```python
from build123d import *

# Parameters (mm, degrees)
SKETCH1_R           = 35
BOSS_EXTRUDE1_DEPTH = 12
SKETCH2_R           = 20.15
CUT_EXTRUDE1_DEPTH  = 5.5
SKETCH3_R           = 2.45
BOSS_EXTRUDE2_DEPTH = 5.5
SKETCH4_R           = 2.5
CUT_EXTRUDE2_DEPTH  = 50.922439844
SKETCH5_R           = 5.5
CUT_EXTRUDE3_DEPTH  = 5
SKETCH6_R           = 2.5
CUT_EXTRUDE4_DEPTH  = 51.931326313
CHAMFER1_SIZE       = 0.5
CHAMFER2_SIZE       = 0.5
CHAMFER3_SIZE       = 0.5


with BuildPart() as part:
    # Sketch1 → Boss-Extrude1 (new body)
    with BuildSketch(Plane(origin=(0, 0, 0), x_dir=(1, 0, 0), z_dir=(0, 1, 0))):
        with Locations(Location((0, 0, 0), (0, 0, 270))):
            Circle(SKETCH1_R)
    extrude(amount=BOSS_EXTRUDE1_DEPTH)

    # Sketch2 → Cut-Extrude1 (cut)
    with BuildSketch(Plane(origin=(0, 12, 0), x_dir=(1, 0, 0), z_dir=(0, 1, 0))):
        with Locations(Location((0, 0, 0), (0, 0, 270))):
            Circle(SKETCH2_R)
    extrude(amount=-CUT_EXTRUDE1_DEPTH, mode=Mode.SUBTRACT)

    # Sketch3 → Boss-Extrude2 (add)
    with BuildSketch(Plane(origin=(0, 6.5, 0), x_dir=(1, 0, 0), z_dir=(0, 1, 0))):
        with Locations(Location((0, -15.75, 0), (0, 0, 270))):
            Circle(SKETCH3_R)
    extrude(amount=BOSS_EXTRUDE2_DEPTH)

    # Sketch4 → Cut-Extrude2 (cut, through all)
    with BuildSketch(Plane(origin=(0, 6.5, 0), x_dir=(1, 0, 0), z_dir=(0, 1, 0))):
        with Locations(Location((11.136931804, 11.136931804, 0), (0, 0, 270))):
            Circle(SKETCH4_R)
        with Locations(Location((11.136931804, -11.136931804, 0), (0, 0, 270))):
            Circle(SKETCH4_R)
        with Locations(Location((-11.136931804, -11.136931804, 0), (0, 0, 270))):
            Circle(SKETCH4_R)
        with Locations(Location((-11.136931804, 11.136931804, 0), (0, 0, 270))):
            Circle(SKETCH4_R)
    extrude(amount=-CUT_EXTRUDE2_DEPTH, mode=Mode.SUBTRACT)

    # Sketch5 → Cut-Extrude3 (cut)
    with BuildSketch(Plane.XZ):
        with Locations(Location((11.136931804, -11.136931804, 0), (0, 0, 270))):
            Circle(SKETCH5_R)
        with Locations(Location((11.136931804, 11.136931804, 0), (0, 0, 270))):
            Circle(SKETCH5_R)
        with Locations(Location((-11.136931804, -11.136931804, 0), (0, 0, 270))):
            Circle(SKETCH5_R)
        with Locations(Location((-11.136931804, 11.136931804, 0), (0, 0, 270))):
            Circle(SKETCH5_R)
    extrude(amount=-CUT_EXTRUDE3_DEPTH, mode=Mode.SUBTRACT)

    # Sketch6 → Cut-Extrude4 (cut, through all)
    with BuildSketch(Plane.XZ):
        with Locations(Location((28.702, 0, 0), (0, 0, 270))):
            Circle(SKETCH6_R)
        with Locations(Location((20.295378834, -20.295378834, 0), (0, 0, 270))):
            Circle(SKETCH6_R)
        with Locations(Location((0, -28.702, 0), (0, 0, 270))):
            Circle(SKETCH6_R)
        with Locations(Location((-20.295378834, -20.295378834, 0), (0, 0, 270))):
            Circle(SKETCH6_R)
        with Locations(Location((-28.702, 0, 0), (0, 0, 270))):
            Circle(SKETCH6_R)
        with Locations(Location((-20.295378834, 20.295378834, 0), (0, 0, 270))):
            Circle(SKETCH6_R)
        with Locations(Location((0, 28.702, 0), (0, 0, 270))):
            Circle(SKETCH6_R)
        with Locations(Location((20.295378834, 20.295378834, 0), (0, 0, 270))):
            Circle(SKETCH6_R)
    extrude(amount=-CUT_EXTRUDE4_DEPTH, mode=Mode.SUBTRACT)

    # Chamfer1
    chamfer1_edges = [part.edges().sort_by_distance(p)[0] for p in [
        (0, 0, -35),
        (-11.136931804, 0, 16.636931804),
        (-11.136931804, 0, -5.636931804),
        (11.136931804, 0, -5.636931804),
        (11.136931804, 0, 16.636931804),
        (28.702, 0, 2.5),
        (20.295378834, 0, -17.795378834),
        (0, 0, -26.202),
        (-20.295378834, 0, -17.795378834),
        (-28.702, 0, 2.5),
        (-20.295378834, 0, 22.795378834),
        (0, 0, 31.202),
        (20.295378834, 0, 22.795378834),
    ]]
    chamfer(chamfer1_edges, length=CHAMFER1_SIZE)

    # Chamfer2
    chamfer2_edges = [part.edges().sort_by_distance(p)[0] for p in [
        (0, 12, -35),
        (0, 12, -20.15),
        (28.702, 12, 2.5),
        (20.295378834, 12, -17.795378834),
        (0, 12, -26.202),
        (-20.295378834, 12, -17.795378834),
        (-28.702, 12, 2.5),
        (-20.295378834, 12, 22.795378834),
        (0, 12, 31.202),
        (20.295378834, 12, 22.795378834),
    ]]
    chamfer(chamfer2_edges, length=CHAMFER2_SIZE)

    # Chamfer3
    chamfer3_edges = [part.edges().sort_by_distance(p)[0] for p in [
        (0, 12, 13.3),
    ]]
    chamfer(chamfer3_edges, length=CHAMFER3_SIZE)


solid = part.part
```
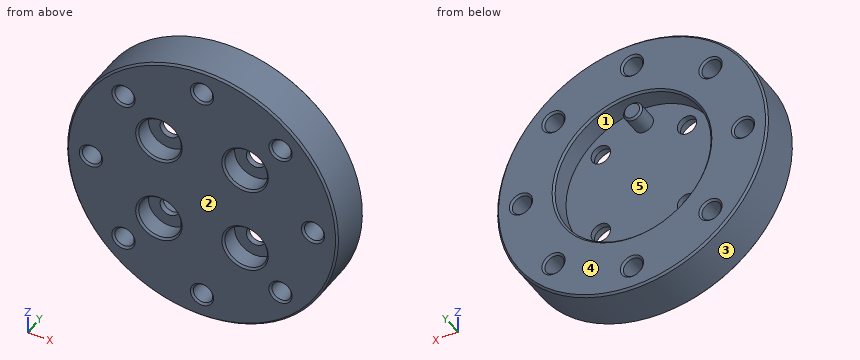
Here's how the part is built. I have some questions about the finished solid (model axes, mm). Face numbers are marked on the shaded views. A direction names the side the tool comes from. Round coordinates to 2 decimals unless told otherwise and drop trailing zeros. Answer as CSV lines item,"result". Start each with the question number.
1. Imagine slicing it at A-A on z = 0. State how many separate pieces and enclosed holes the cut face has, plus the area to 3 significant figures.
2. If we mould it in two halves opening along X, with no side actions, what happens to the marked faces 1, 2 and 3? For each: pulls with the +X half, pulls with the -X half, needs draft (parallel to the pull), parting line crosses it, or undercut.
3. I'm going to push flat-ended pins straight in: P1, Ø1.5, axis at x = 7, y = 10, coming from the -Z side; P2, Ø2, axis at x = -4.5, y = 5, coming from the -Z side; P3, Ø5.5, axis at x = -12.5, z = -13, coming from the -Y side; P4, Ø4.5, axis at x = 0, z = 28.702, coming from the -Y side. Where does each tip first touch, or does it pass through?
4. For the marked faces 4 and 5, which set-ups out of +Z, -Z, +X, -X, +Y, -Y let a thin tool reach every point of the face, with its end or its side?
5. I need wall thicknesses on probe 1 along X at (y, z) = (2, -13.5); probe 2 along Z at (x, y) = (-13, 4.25); probe 3 along X at (y, z) = (7.5, 0). Which ranges of each line are inside material? Lowest first, please. Write a range as from..to.
Solution:
1,separate pieces,"3"
1,enclosed holes,"0"
1,area,"497 mm²"
2,face 1,"undercut"
2,face 2,"needs draft"
2,face 3,"parting line crosses it"
3,P1,"z = -34.44"
3,P2,"z = -34.82"
3,P3,"y = 5"
3,P4,"through"
4,face 4,"+Z, -Z, +X, -X, +Y"
4,face 5,"+Y"
5,probe 1,"-32.29..-16.1, -6.17..6.17, 16.1..32.29"
5,probe 2,"-32.5..-16.31, -5.96..5.96, 16.31..32.5"
5,probe 3,"-35..-31.2, -26.2..-20.15, 20.15..26.2, 31.2..35"
